Can you work these out from the model? Positions are in its coordinate system, mm. A direction names the side the tool comes from. Give positions to 0.01 mm unless a question says otherwise; leave off trailing zeros. Write each loop counter-clockwise with the first axis right and the second up, starting at its lowest first coordinate (ties: lowest second). Pieces come first, ordered by that corner, then holes. Notation, with made-up numbers: M 77.25,53 L 83.25,53 A27 cw 83.25,69 Z; hole C -31.75,70 d2. An arc over 180 degrees is marked long. Write each question's results on one line, items separated by ' | '.
from build123d import *

# Parameters (mm, degrees)
SKETCH1_W           = 27
SKETCH1_H           = 63.1
SKETCH1_R           = 2.5
BOSS_EXTRUDE1_DEPTH = 3
SKETCH2_W           = 27
SKETCH2_H           = 45.1
BOSS_EXTRUDE2_DEPTH = 43.66
CUT_EXTRUDE1_DEPTH  = 28
SKETCH3_8_W         = 42.1
SKETCH3_8_H         = 42.16
SKETCH3_8_R         = 2
CUT_EXTRUDE2_DEPTH  = 26
FILLET4_R           = 1
SKETCH6_W           = 6.985
SKETCH6_H           = 7.95
CUT_EXTRUDE3_DEPTH  = 1.5
SKETCH3_9_R         = 2
CUT_EXTRUDE4_DEPTH  = 28


with BuildPart() as part:
    # Sketch1 → Boss-Extrude1 (new body)
    with BuildSketch(Plane(origin=(0, 0, 0), x_dir=(1, 0, 0), z_dir=(0, 1, 0))):
        with Locations((13.5, 31.55)):
            Rectangle(SKETCH1_W, SKETCH1_H)
        with Locations((3.5, 58.1)):
            Circle(SKETCH1_R, mode=Mode.SUBTRACT)
        with Locations((23.5, 58.1)):
            Circle(SKETCH1_R, mode=Mode.SUBTRACT)
    extrude(amount=BOSS_EXTRUDE1_DEPTH)

    # Sketch2 → Boss-Extrude2 (add)
    with BuildSketch(Plane(origin=(0, 3, 0), x_dir=(1, 0, 0), z_dir=(0, 1, 0))):
        with Locations((13.5, 22.55)):
            Rectangle(SKETCH2_W, SKETCH2_H)
    extrude(amount=BOSS_EXTRUDE2_DEPTH)

    # Sketch3 → Cut-Extrude1 (cut, through all)
    with BuildSketch(Plane.ZY):
        with BuildLine():
            Line((-10.38, 45.16), (-34.72, 45.16))
            Line((-34.72, 45.16), (-34.72, 39.61))
            ThreePointArc((-34.72, 39.61), (-35.695334419, 37.255334419), (-38.05, 36.28))
            Line((-38.05, 36.28), (-43.6, 36.28))
            Line((-43.6, 36.28), (-43.6, 11.88))
            Line((-43.6, 11.88), (-38.05, 11.88))
            ThreePointArc((-38.05, 11.88), (-35.695334419, 10.904665581), (-34.72, 8.55))
            Line((-34.72, 8.55), (-34.72, 3))
            Line((-34.72, 3), (-10.38, 3))
            Line((-10.38, 3), (-10.38, 8.55))
            ThreePointArc((-10.38, 8.55), (-9.404665581, 10.904665581), (-7.05, 11.88))
            Line((-7.05, 11.88), (-1.5, 11.88))
            Line((-1.5, 11.88), (-1.5, 36.28))
            Line((-1.5, 36.28), (-7.05, 36.28))
            ThreePointArc((-7.05, 36.28), (-9.404665581, 37.255334419), (-10.38, 39.61))
            Line((-10.38, 39.61), (-10.38, 45.16))
        make_face()
    extrude(amount=-CUT_EXTRUDE1_DEPTH, mode=Mode.SUBTRACT)

    # Sketch3<8> → Cut-Extrude2 (cut)
    with BuildSketch(Plane.ZY):
        with Locations((-22.55, 24.08)):
            Rectangle(SKETCH3_8_W, SKETCH3_8_H)
        with Locations((-38.05, 8.55)):
            Circle(SKETCH3_8_R, mode=Mode.SUBTRACT)
        with Locations((-7.05, 39.61)):
            Circle(SKETCH3_8_R, mode=Mode.SUBTRACT)
        with Locations((-7.05, 8.55)):
            Circle(SKETCH3_8_R, mode=Mode.SUBTRACT)
        with Locations((-38.05, 39.61)):
            Circle(SKETCH3_8_R, mode=Mode.SUBTRACT)
    extrude(amount=-CUT_EXTRUDE2_DEPTH, mode=Mode.SUBTRACT)

    # Fillet4
    fillet4_edges = [part.edges().sort_by_distance(p)[0] for p in [
        (0, 45.16, -22.55),
        (0, 24.08, -1.5),
        (0, 3, -22.55),
        (0, 24.08, -43.6),
    ]]
    fillet(fillet4_edges, radius=FILLET4_R)

    # Sketch6 → Cut-Extrude3 (cut)
    with BuildSketch(Plane(origin=(0, 46.66, 0), x_dir=(1, 0, 0), z_dir=(0, 1, 0))):
        with Locations((23.5075, 22.675)):
            Rectangle(SKETCH6_W, SKETCH6_H)
    extrude(amount=-CUT_EXTRUDE3_DEPTH, mode=Mode.SUBTRACT)

    # Sketch3<9> → Cut-Extrude4 (cut, through all)
    with BuildSketch(Plane.ZY):
        with Locations((-38.05, 39.61)):
            Circle(SKETCH3_9_R)
        with Locations((-7.05, 39.61)):
            Circle(SKETCH3_9_R)
        with Locations((-7.05, 8.55)):
            Circle(SKETCH3_9_R)
        with Locations((-38.05, 8.55)):
            Circle(SKETCH3_9_R)
    extrude(amount=-CUT_EXTRUDE4_DEPTH, mode=Mode.SUBTRACT)


solid = part.part
Item 1: I want a section at A-A, the plane x = 3.5. Please give me the cut outline in (y, z), and give its area (3 significant figures).
Geometry says:
outline: M 0,-63.1 L 3,-63.1 L 3,-60.6 L 0,-60.6 Z; M 0,-55.6 L 3,-55.6 L 3,-45.1 L 46.66,-45.1 L 46.66,0 L 0,0 Z; hole M 3,-43.6 L 45.16,-43.6 L 45.16,-1.5 L 3,-1.5 Z | area: 368 mm2
Item 2: I want a section at D-D, the plane x = 15. Please give me the cut outline in (y, z), and give its area (3 significant figures).
Geometry says:
outline: M 0,-63.1 L 3,-63.1 L 3,-45.1 L 46.66,-45.1 L 46.66,0 L 0,0 Z; hole M 3,-43.6 L 45.16,-43.6 L 45.16,-1.5 L 3,-1.5 Z | area: 383 mm2
Item 3: I'm going to push flat-ended pins straight in: pin 1 (5.5 mm diameter, centred on x = 13, z = -52.5, fed in from +Y); pin 2 (1.2 mm diameter, centred on y = 45.5, z = -23.5, fed in from +X) (3 decimals); pin 3 (1.2 mm diameter, centred on x = 22, y = 45.5, fed in from -Z). Where does each tip first touch, or does it pass through?
Geometry says:
pin 1: stops at y = 3 | pin 2: stops at x = 20.015 | pin 3: stops at z = -45.1
Item 4: For faces 1 (the face through (14, 45.16, -22)), 2 (the face through (13, 3, -54)), 3 (the face through (26.49, 10.93, -35.72)), which set-ups out of +Z, -Z, +X, -X, +Y, -Y let a thin tool reach every point of the face, with its end or its side?
Geometry says:
face 1: -X | face 2: -Z, +X, -X, +Y | face 3: +X, -X
Item 5: If I drill on line 1 (X direction, y = 2.2, z = -58.1); line 2 (Y direction, x = 26.3, z = -7.05); line 3 (Y direction, x = 5.75, z = -16), over which ranges is the centre line in solid material (lowest first)? Write a range as from..to.
Geometry says:
line 1: x = 0..1, 6..21, 26..27 | line 2: y = 0..6.55, 10.55..11.88, 36.28..37.61, 41.61..46.66 | line 3: y = 0..3, 45.16..46.66
Item 6: I want a section at B-B, the plane y = 43. Please give me the cut outline in (x, z).
Geometry says:
outline: M 0,-45.1 L 27,-45.1 L 27,-34.72 L 26,-34.72 L 26,-43.6 L 1,-43.6 A1 ccw 0,-44.6 Z; M 0,-0.5 A1 ccw 1,-1.5 L 26,-1.5 L 26,-10.38 L 27,-10.38 L 27,0 L 0,0 Z
Item 7: I want a section at C-C, the plane z = -24. Please give me the cut outline in (x, y) (3 decimals), and give its area (3 significant figures).
Geometry says:
outline: M 0,0 L 27,0 L 27,3 L 1,3 A1 ccw 0,2 Z; M 0,46.16 A1 ccw 1,45.16 L 20.015,45.16 L 20.015,46.66 L 0,46.66 Z | area: 111 mm2
Item 8: Thinking about a two-plate mould opening in X: for faces 4 (the face through (26.49, 37.23, -9.38)), 5 (the face through (4.84, 1.48, -60.21)), 6 (the face through (26, 41, -40)), which applies, +X half, -X half, draft (parallel to the pull), parting line (faces both ways), or undercut?
Geometry says:
face 4: draft | face 5: undercut | face 6: -X half
